The drawing under review shows one solid part. Ordinate dimensions are in mm from its lowest x, y, z. Round coordinates to 2 decimals unless told otherwise and drop trailing zeros. Write each loop counter-clockwise with the first axis right and the second up, starting at its lowest first coordinate (ties: lowest second). Pieces come first, ordered by that corner, then holes. Notation, with made-up numbers: (-40, 65.25) - (-16, 65.25) arc R17 ccw to (-16, 78.25) - close; hole circle Ø5 at (58.5, 52.25). An arc over 180 degrees is marked (long way). One line per question, with ' | ' between items. Start each with the question number.
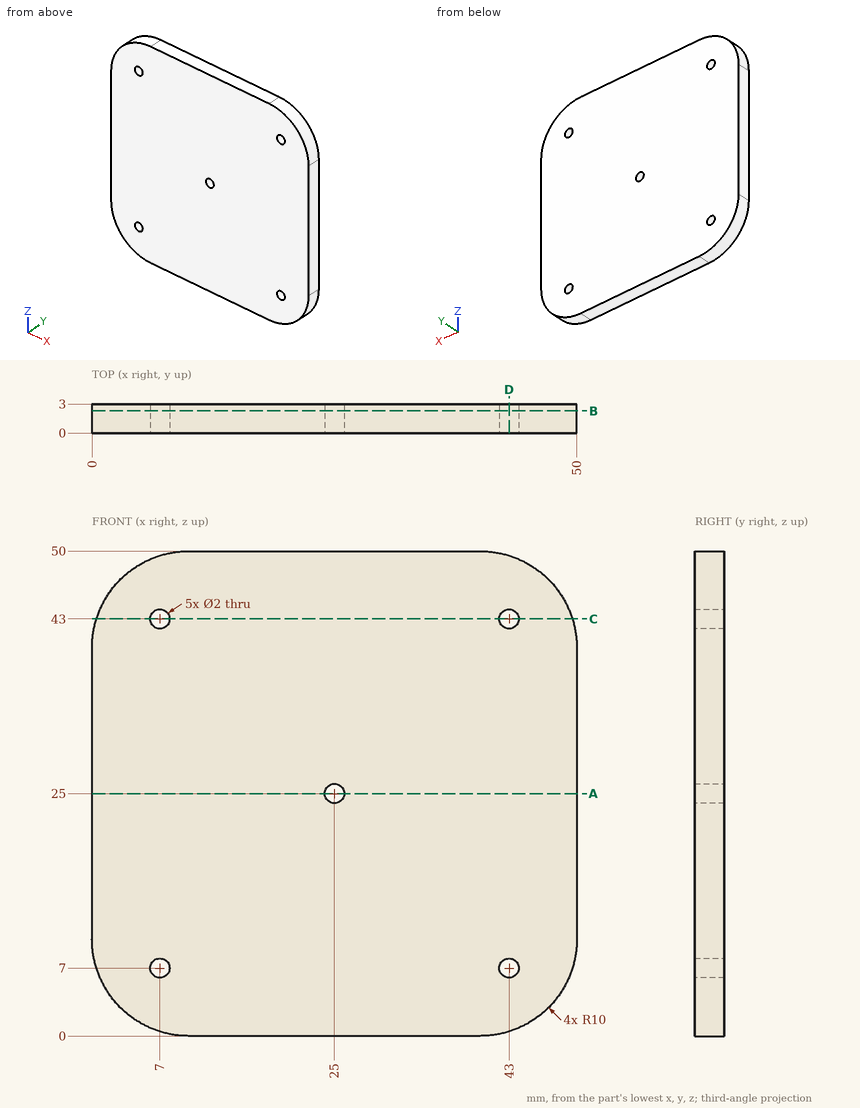
1. Add section D-D, the plane x = 43. Write out the cut boundary in (y, z), then the cut area to 3 significant figures.
2. Add section B-B, the plane y = 2.3. Write out the cut boundary in (x, z), then the cut area to 3 significant figures.
3. Add section C-C, the plane z = 43. Write out the cut boundary in (x, y).
4. Wall thickness on line 1 along X through (y, z) = (2.25, 43); line 2 along Z through (x, y) = (3, 2.75): over which ranges is each line inside the solid? List them lowest first. Write a range as [from, to].
5. Add section A-A, the plane z = 25. Write out the cut boundary in (x, y).
Geometry check:
1) outline: (0, 0.46) - (3, 0.46) - (3, 6) - (0, 6) - close; (0, 8) - (3, 8) - (3, 42) - (0, 42) - close; (0, 44) - (3, 44) - (3, 49.54) - (0, 49.54) - close | area: 135 mm2
2) outline: (0, 10) arc R10 ccw to (10, 0) - (40, 0) arc R10 ccw to (50, 10) - (50, 40) arc R10 ccw to (40, 50) - (10, 50) arc R10 ccw to (0, 40) - close; hole circle Ø2 at (7, 7); hole circle Ø2 at (7, 43); hole circle Ø2 at (25, 25); hole circle Ø2 at (43, 7); hole circle Ø2 at (43, 43) | area: 2,400 mm2
3) outline: (0.46, 0) - (6, 0) - (6, 3) - (0.46, 3) - close; (8, 0) - (42, 0) - (42, 3) - (8, 3) - close; (44, 0) - (49.54, 0) - (49.54, 3) - (44, 3) - close
4) line 1: x = [0.46, 6], [8, 42], [44, 49.54] | line 2: z = [2.86, 47.14]
5) outline: (0, 0) - (24, 0) - (24, 3) - (0, 3) - close; (26, 0) - (50, 0) - (50, 3) - (26, 3) - close
